For this review, use the dimensioned drawing (mm, ordinates from the lowest corner) and the shaded views. Give positions to 0.01 mm unless a question says otherwise; leave off trailing zeros. Order: outer loops, then holes, each group sorted by start corner. A loop starts at its lowest first (then second) coordinate and runs counter-clockwise, first axis right, second up.
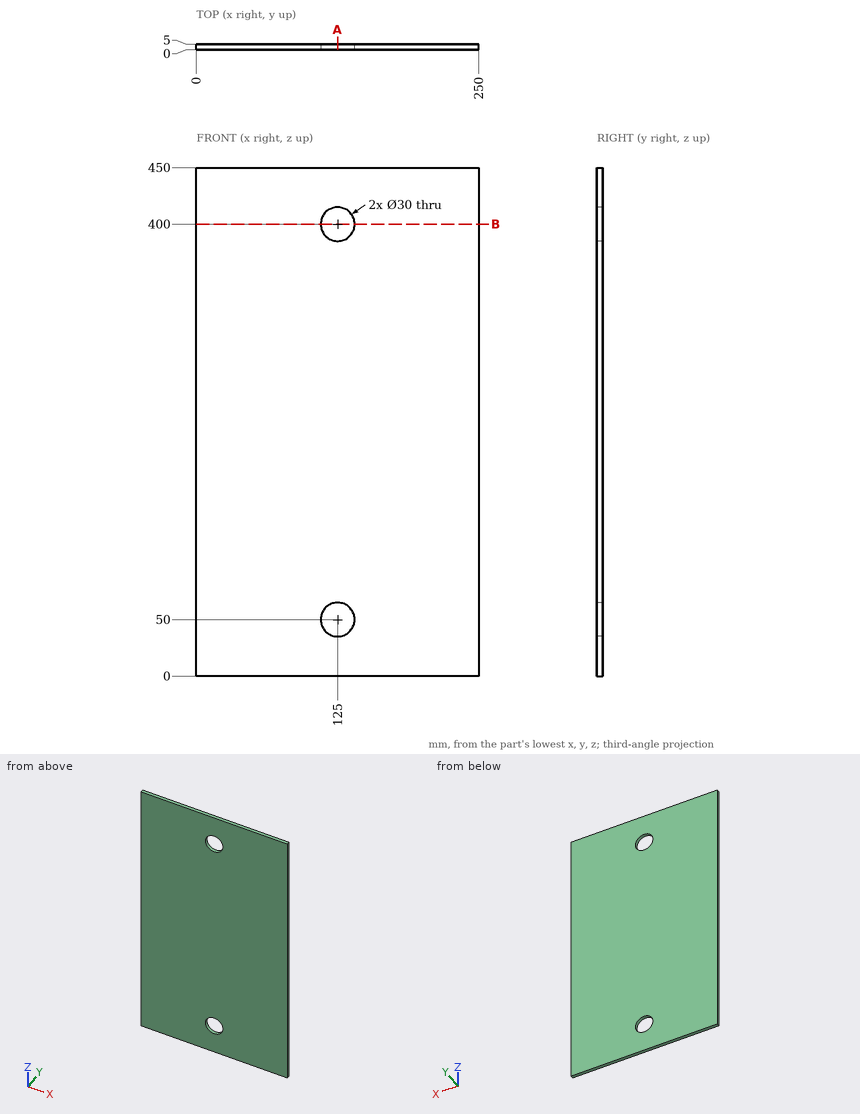
1. Take a section at B-B (z = 400). Write out the cut boundary in (x, y).
2. Take a section at A-A (x = 125). Write out the cut boundary in (y, z), and give its area (3 significant figures).
3. To check wall thickness, follow line 1 (Z direction, x = 125, y = 2.7); line 2 (X direction, y = 2.05, z = 388). State the ranges of each line that lie inside material, in increasing order.
Answer:
1. outline: (0, 0) - (110, 0) - (110, 5) - (0, 5) - close; (140, 0) - (250, 0) - (250, 5) - (140, 5) - close
2. outline: (0, 0) - (5, 0) - (5, 35) - (0, 35) - close; (0, 65) - (5, 65) - (5, 385) - (0, 385) - close; (0, 415) - (5, 415) - (5, 450) - (0, 450) - close
2. area: 1,950 mm2
3. line 1: z = 0 to 35, 65 to 385, 415 to 450
3. line 2: x = 0 to 116, 134 to 250
